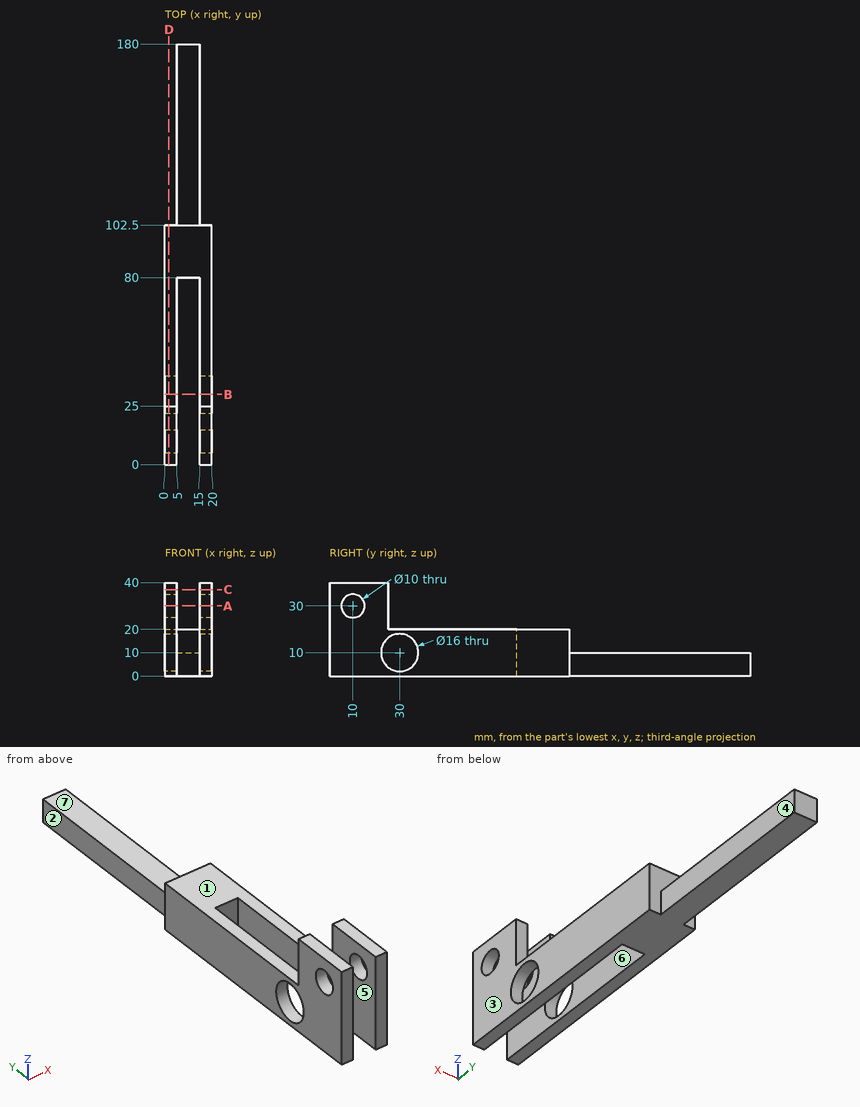
Source: three-view drawing plus pictorial views. Frame: mm from the lowest corner of the part. A direction names the side the tool comes from. Give positions to 0.01 mm unless a question says otherwise; leave off trailing zeros. Order: outer loops, then holes, each group sorted by start corner. A loop starts at its lowest first (then second) coordinate and runs counter-clockwise, first axis right, second up. Notation, with made-up numbers: (41, 69.25) - (69, 69.25) arc R29 cw to (69, 108.25) - close; hole circle Ø4 at (47, 67). An arc over 180 degrees is marked (long way). Put each result on its own line as item: value.
Item 1: Section query C-C, the plane z = 37. Return loops of the section in (x, y), then the cut area to 3 significant figures.
Found:
outline: (0, 0) - (5, 0) - (5, 25) - (0, 25) - close; (15, 0) - (20, 0) - (20, 25) - (15, 25) - close
area: 250 mm^2
Item 2: Access query for the marked faces 1, 2 and 3. Directions: +Z, -Z, +X, -X, +Y, -Y. A direction counts if a zero-diameter tool reaches every point of the face in a straight line with its end or side. Return the directions, or none.
Found:
face 1: +Z, +X, -X, +Y
face 2: +Z, -Z, -X, +Y
face 3: +Z, -Z, +X, +Y, -Y
Item 3: Draft query along X for the marked faces 4, 5, 6 and 7. Return one class per face: +X half, -X half, draft (parallel to the pull), parting line (faces both ways), or undercut.
Found:
face 4: +X half
face 5: undercut
face 6: undercut
face 7: draft
Item 4: Section query B-B, the plane y = 30. Return loops of the section in (x, z).
Found:
outline: (0, 0) - (5, 0) - (5, 2) - (0, 2) - close; (0, 18) - (5, 18) - (5, 20) - (0, 20) - close; (15, 0) - (20, 0) - (20, 2) - (15, 2) - close; (15, 18) - (20, 18) - (20, 20) - (15, 20) - close
Item 5: Section query A-A, the plane z = 30. Return loops of the section in (x, y).
Found:
outline: (0, 0) - (5, 0) - (5, 5) - (0, 5) - close; (0, 15) - (5, 15) - (5, 25) - (0, 25) - close; (15, 0) - (20, 0) - (20, 5) - (15, 5) - close; (15, 15) - (20, 15) - (20, 25) - (15, 25) - close
Item 6: Ray query, L1, parallel to Y at x = 2.2, z = 30; L2, parallel to Y at x = 2.95, z = 10; L3, parallel to X at y = 18, z = 8. Return the intervals inside material, ascending. Write a range as from..to.
Found:
L1: y = 0..5, 15..25
L2: y = 0..22, 38..102.5
L3: x = 0..5, 15..20
Item 7: Contact query for flat-ended pins moving along their axis: pin 1 (6 mm diameter, centred on x = 11, y = 78, fed in from +Z); pin 2 (8 mm diameter, centred on x = 11, y = 139.5, fed in from +Z); pin 3 (2.5 mm diameter, centred on x = 17, z = 31, fed in from +Y). Output: stop coordinate, or through.
Found:
pin 1: stops at z = 20
pin 2: stops at z = 10
pin 3: stops at y = 25
Item 8: Section query D-D, the plane x = 1.75. Return loops of the section in (y, z).
Found:
outline: (0, 0) - (102.5, 0) - (102.5, 20) - (25, 20) - (25, 40) - (0, 40) - close; hole circle Ø10 at (10, 30); hole circle Ø16 at (30, 10)
